```python
from build123d import *

# Parameters (mm, degrees)
F0_W     = 101.05566
F0_H     = 29.790164
F1_DEPTH = 63.5
F2_R     = 22.602142
F3_DEPTH = 25.4
F4_R     = 16.601085
F5_DEPTH = 55.191165


with BuildPart() as f1:
    # F0 (on Top) → F1 (new body)
    with BuildSketch(Plane.XY):
        Rectangle(F0_W, F0_H)
    extrude(amount=F1_DEPTH)

    # F2 (on face) → F3 (join)
    with BuildSketch(Plane.XZ.offset(14.895082)):
        with Locations((0, 32.410629)):
            Circle(F2_R)
    extrude(amount=F3_DEPTH)

    # F4 (on face) → F5 (cut, through all)
    with BuildSketch(Plane.XZ.offset(40.295082)):
        with Locations((0, 32.410629)):
            Circle(F4_R)
    extrude(amount=-F5_DEPTH, mode=Mode.SUBTRACT)


solid = f1.part
```
Source: CAD feature listing. Evaluate the final solid. Frame: model axes, mm. A direction names the side the tool comes from. Round coordinates to 2 decimals unless told otherwise and drop trailing zeros. Loops run counter-clockwise (first coordinate to the right, second up) from the corner with the lowest first, then second, coordinate; pieces in that order, holes last.
(1) Section query B-B (z = 47). Output: boundary loops of the cut face in (x, y), and give its area (3 significant figures).
From the geometry:
outline: (-50.53, -14.9) - (-17.26, -14.9) - (-17.26, -40.3) - (-7.92, -40.3) - (-7.92, 14.9) - (-50.53, 14.9) - close; (7.92, -40.3) - (17.26, -40.3) - (17.26, -14.9) - (50.53, -14.9) - (50.53, 14.9) - (7.92, 14.9) - close
area: 3,010 mm2
(2) Access query for faces 1 (the flat face through (-23, -14.895, 31)), 2 (the flat face through (-12, 14.895, 45)). Directions: +Z, -Z, +X, -X, +Y, -Y. A direction counts if a zero-diameter tool reaches every point of the face in a straight line with its end or side. Return the directions, or none.
From the geometry:
face 1: -Y
face 2: +Z, -Z, +X, -X, +Y
(3) Section query A-A (x = 3). Output: boundary loops of the cut face in (y, z), and give its area (3 significant figures).
From the geometry:
outline: (-40.3, 10.01) - (-14.9, 10.01) - (-14.9, 0) - (14.9, 0) - (14.9, 16.08) - (-40.3, 16.08) - close; (-40.3, 48.74) - (14.9, 48.74) - (14.9, 63.5) - (-14.9, 63.5) - (-14.9, 54.81) - (-40.3, 54.81) - close
area: 1,230 mm2
(4) Section query D-D (x = -32). Output: boundary loops of the cut face in (y, z).
From the geometry:
outline: (-14.9, 0) - (14.9, 0) - (14.9, 63.5) - (-14.9, 63.5) - close
(5) Material intervals for probe 1 along Z at (x, y) = (0, -22.5); probe 2 along Z at (x, y) = (0, -11.5); probe 3 along X at (y, z) = (-4, 33), sorted ascending.
From the geometry:
probe 1: z = 9.81 to 15.81, 49.01 to 55.01
probe 2: z = 0 to 15.81, 49.01 to 63.5
probe 3: x = -50.53 to -16.59, 16.59 to 50.53
(6) Pull-direction query (Z, two-part tool) for faces 3 (the cylindrical face through (-3.599, -13.086, 16.204)), 4 (the flat face through (-1, 0, 0)), 5 (the cylindrical face through (-2.94, -27.42, 54.82)); classes: +Z half, -Z half, draft (parallel to the pull), parting line (faces both ways), or undercut.
From the geometry:
face 3: undercut
face 4: -Z half
face 5: parting line
(7) Contact query for flat-ended pins moving along their axis: pin 1 Ø6 at (y, z) = (-32.5, 49) entering from -X; pin 2 Ø6 at (x, z) = (23.5, 45.5) entering from -Y. Output: stop coordinate, or through.
From the geometry:
pin 1: stops at x = -18.06
pin 2: stops at y = -14.9
(8) Section query C-C (y = 1). Output: boundary loops of the cut face in (x, z), and give its area (3 significant figures).
From the geometry:
outline: (-50.53, 0) - (50.53, 0) - (50.53, 63.5) - (-50.53, 63.5) - close; hole circle Ø33.2 at (0, 32.41)
area: 5,550 mm2
